Can you work these out from the model? Positions are in its coordinate system, mm. A direction names the side the tool comes from. Coordinates: 2 decimals unless noted, no trailing zeros. Write each loop counter-clockwise with the first axis right and the second up, starting at its lowest first coordinate (ties: lowest second). Pieces come first, ordered by that corner, then holes.
```python
from build123d import *

# Parameters (mm, degrees)
F0_W     = 10
F0_H     = 10
F1_DEPTH = 25
F2_W     = 22.988717
F2_H     = 25
F3_DEPTH = 5
F4_W     = 6.904623
F4_H     = 25.005924
F5_DEPTH = 25.8


with BuildPart() as f1:
    # F0 (on Top) → F1 (new body)
    with BuildSketch(Plane.XY):
        with Locations((10, 25)):
            Rectangle(F0_W, F0_H)
        with Locations((25, 25)):
            Rectangle(F0_W, F0_H)
        with Locations((25, 10)):
            Rectangle(F0_W, F0_H)
        with Locations((10, 10)):
            Rectangle(F0_W, F0_H)
    extrude(amount=F1_DEPTH)

    # F2 (on Top) → F3 (join)
    with BuildSketch(Plane.XY):
        with Locations((16.494358, 17.5)):
            Rectangle(F2_W, F2_H)
    extrude(amount=F3_DEPTH)

    # F4 (on Top) → F5 (join)
    with BuildSketch(Plane.XY):
        with Locations((26.778734, 17.541469)):
            Rectangle(F4_W, F4_H)
    extrude(amount=-F5_DEPTH)


solid = f1.part
```
1. If we section it at C-C, the plane y = 16.5: List the corners of the cut face in (x, z) for me, plus the area to 3 significant figures.
2. We'd pull the mould along Y, two halves only. Please class faces 1 (the face through (10, 15, 15)), 2 (the face through (15, 18, 0)), 3 (the face through (14.5, 30, 12.3)): released by +Y, released by -Y, zero draft, split by the parting line, or undercut.
3. Which directions (+Z, -Z, +X, -X, +Y, -Y) give clear straight access to the entire face, cutting with the end or side of a thin tool? Please do faces 4 (the face through (25, 10, 25)), 5 (the face through (5, 10, 15)), 6 (the face through (30, 10, 12)), 7 (the face through (23.326, 17, -13)), 8 (the face through (15, 25, 15)).
4. I'm going to push flat-ended pins straight in: P1, Ø1, axis at x = 20.5, z = 9, coming from the +Y side; P2, Ø3, axis at x = 15.5, y = 17.5, coming from the -Z side; P3, Ø11, axis at y = 12, z = 8.5, coming from the +X side; P4, Ø5.5, axis at x = 26.5, y = 16.5, coming from the +Z side. Where does each tip first touch, or does it pass through?
5. If we section it at A-A, the plane z = 16.5: List the corners of the cut face in (x, y) for me.
6. If we section it at B-B, the plane x = 12.75: List the corners of the cut face in (y, z) for me, plus the area to 3 significant figures.
7. If I drill on L1, parallel to X at y = 12.25, z = 7; L2, parallel to Z at x = 21.25, y = 27.5, over which ranges is the centre line in solid material (lowest first)?
Answers:
1. outline: (5, 0) - (23.33, 0) - (23.33, -25.8) - (30.23, -25.8) - (30.23, 0) - (27.99, 0) - (27.99, 5) - (5, 5) - close
1. area: 293 mm2
2. face 1: undercut
2. face 2: zero draft
2. face 3: released by +Y
3. face 4: +Z, +X, -X, +Y, -Y
3. face 5: +Z, -Z, -X, +Y, -Y
3. face 6: +Z, +X, +Y, -Y
3. face 7: -Z, -X, +Y, -Y
3. face 8: +Z, +Y, -Y
4. P1: stops at y = 30
4. P2: stops at z = 0
4. P3: stops at x = 30
4. P4: stops at z = 25
5. outline: (5, 5) - (15, 5) - (15, 15) - (5, 15) - close; (5, 20) - (15, 20) - (15, 30) - (5, 30) - close; (20, 5) - (30, 5) - (30, 15) - (20, 15) - close; (20, 20) - (30, 20) - (30, 30) - (20, 30) - close
6. outline: (5, 0) - (30, 0) - (30, 25) - (20, 25) - (20, 5) - (15, 5) - (15, 25) - (5, 25) - close
6. area: 525 mm2
7. L1: x = 5 to 15, 20 to 30
7. L2: z = 0 to 25
